Verification items for the finished model (mm, model axes). A direction names the side the tool comes from. Give positions to 0.01 mm unless a question says otherwise; leave off trailing zeros. Loops run counter-clockwise (first coordinate to the right, second up) from the corner with the lowest first, then second, coordinate; pieces in that order, holes last. Notation, with made-up numbers: M 15,1.25 L 59,1.25 A21 ccw 59,10.25 Z; hole C 51.25,-19.5 d7. An arc over 180 degrees is marked long. Use a Markdown table: item, result.
from build123d import *

# Parameters (mm, degrees)
SALIENTE_EXTRUIR1_DEPTH     = 120
CORTAR_EXTRUIR4_DEPTH       = 118
CORTAR_EXTRUIR4_DEPTH_BACK  = 26
CROQUIS2_W                  = 62.5
CROQUIS2_H                  = 46
CORTAR_EXTRUIR10_DEPTH      = 30
CORTAR_EXTRUIR10_DEPTH_BACK = 41
CROQUIS3_R                  = 16.752869439


with BuildPart() as part:
    # Croquis1 → Saliente-Extruir1 (new body)
    with BuildSketch(Plane.XY):
        Polygon((-124.610735746, 44.963996627), (-74.610735746, 44.963996627), (-74.610735746, -5.036003373), (-78.610735746, -5.036003373), (-78.610735746, 40.963996627), (-124.610735746, 40.963996627), align=None)
    extrude(amount=SALIENTE_EXTRUIR1_DEPTH)

    # Croquis2 → Cortar-Extruir4 (cut, two sides: drawn at the far end of the back side and taken through both)
    with BuildSketch(Plane.ZY.offset(78.610735746).offset(-CORTAR_EXTRUIR4_DEPTH_BACK)):
        with Locations((31.25, 17.963996627)):
            Rectangle(CROQUIS2_W, CROQUIS2_H)
    extrude(amount=CORTAR_EXTRUIR4_DEPTH + CORTAR_EXTRUIR4_DEPTH_BACK, mode=Mode.SUBTRACT)

    # Croquis3 → Cortar-Extruir10 (cut, two sides: drawn at the far end of the back side and taken through both)
    with BuildSketch(Plane.XZ.offset(-40.963996627).offset(-CORTAR_EXTRUIR10_DEPTH_BACK)):
        with Locations(Location((-101.610735746, 97, 0), (0, 0, 270))):
            Circle(CROQUIS3_R)
    extrude(amount=CORTAR_EXTRUIR10_DEPTH + CORTAR_EXTRUIR10_DEPTH_BACK, mode=Mode.SUBTRACT)


solid = part.part
(1) Cross-section at A-A on z = 97. Record the cut outline in (x, y).
Results below:
| item | result |
|---|---|
| outline | M -124.61,40.96 L -118.36,40.96 L -118.36,44.96 L -124.61,44.96 Z; M -84.86,40.96 L -78.61,40.96 L -78.61,-5.04 L -74.61,-5.04 L -74.61,44.96 L -84.86,44.96 Z |
(2) Cross-section at C-C on z = 10. Record the cut outline in (x, y), then the cut area to 3 significant figures.
Results below:
| item | result |
|---|---|
| outline | M -124.61,40.96 L -74.61,40.96 L -74.61,44.96 L -124.61,44.96 Z |
| area | 200 mm^2 |
(3) Set-up check for faces 1 (the flat face through (-78.611, 18, 91)), 2 (the flat face through (-77, 18, 62.5)), 3 (the flat face through (-77, -5.036, 91)): record each of +Z, -Z, +X, -X, +Y, -Y from which the full face is reachable in a straight line by a thin tool's end or side.
Results below:
| item | result |
|---|---|
| face 1 | +Z, -Z, -X, -Y |
| face 2 | -Z, +X, -X, -Y |
| face 3 | +Z, -Z, +X, -X, -Y |
(4) Draft check along Z on faces 4 (the flat face through (-99, 40.964, 46)), 5 (the cylindrical face through (-87.485, 42.992, 87.994)), 6 (the flat face through (-77, 31, 120)). Enter one of: +Z half, -Z half, draft (parallel to the pull), parting line (faces both ways), or undercut.
Results below:
| item | result |
|---|---|
| face 4 | draft |
| face 5 | undercut |
| face 6 | +Z half |
(5) Material ranges on line 1 (X direction, y = 43.05, z = 97); line 2 (Y direction, x = -107, z = 114.5); line 3 (Z direction, x = -78, y = 0), recorded low to high.
Results below:
| item | result |
|---|---|
| line 1 | -124.61 to -118.36, -84.86 to -74.61 |
| line 2 | 40.96 to 44.96 |
| line 3 | 62.5 to 120 |
(6) Gauge pin test, flat ends, axial feed: P1, Ø10, axis at x = -113, z = 36, coming from the -Y side; P2, Ø4.5, axis at x = -77.5, y = 19.5, coming from the -Z side; P3, Ø23, axis at y = 27, z = 86, coming from the -X side. Record the tip position at first contact, or that the pin passes through.
Results below:
| item | result |
|---|---|
| P1 | y = 40.96 |
| P2 | z = 62.5 |
| P3 | x = -78.61 |
(7) Cross-section at B-B on y = 37. Record the cut outline in (x, z), then the cut area to 3 significant figures.
Results below:
| item | result |
|---|---|
| outline | M -78.61,62.5 L -74.61,62.5 L -74.61,120 L -78.61,120 Z |
| area | 230 mm^2 |
